```python
from build123d import *

# Parameters (mm, degrees)
SIDEBUMPERS_START       = -58.795147929
SIDEBUMPERS_OUTLINE_W   = 5.08
SIDEBUMPERS_OUTLINE_H   = 12.7
SIDEBUMPERS_DEPTH       = 21
SIDEBUMPERS_START_2     = -79.295147929
SIDEBUMPERS_2_OUTLINE_W = 5.08
SIDEBUMPERS_2_OUTLINE_H = 2.54
SIDEBUMPERS_2_DEPTH     = 62
SKETCH3_W               = 20.5
SKETCH3_H               = 5.08
CUT_EXTRUDE1_DEPTH      = 5.08
SKETCH5_W               = 21
SKETCH5_H               = 5.08
BOSS_EXTRUDE1_DEPTH     = 3
SKETCH8_W               = 41.5
SKETCH8_H               = 5.08
BOSS_EXTRUDE3_DEPTH     = 12
FILLET2_R               = 12
SKETCH9_W               = 4
SKETCH9_H               = 8.7
CUT_EXTRUDE5_DEPTH      = 5.08


# Read off the part's stored shape, not the designer's step: SideBumpers
with BuildPart() as part:
    # SideBumpers outline → SideBumpers (new body)
    with BuildSketch(Plane.YZ.offset(SIDEBUMPERS_START)):
        with Locations((-9.174171779, 10.734849265)):
            Rectangle(SIDEBUMPERS_OUTLINE_W, SIDEBUMPERS_OUTLINE_H)
    extrude(amount=SIDEBUMPERS_DEPTH)

    # SideBumpers 2 outline → SideBumpers 2 (add)
    with BuildSketch(Plane.YZ.offset(SIDEBUMPERS_START_2)):
        with Locations((-9.174171779, 5.654849265)):
            Rectangle(SIDEBUMPERS_2_OUTLINE_W, SIDEBUMPERS_2_OUTLINE_H)
    extrude(amount=SIDEBUMPERS_2_DEPTH)

    # Sketch3 → Cut-Extrude1 (cut)
    with BuildSketch(Plane(origin=(0, 0, 4.384849265), x_dir=(-1, 0, 0), z_dir=(0, 0, -1))):
        with Locations((27.545147929, -9.174171779)):
            Rectangle(SKETCH3_W, SKETCH3_H)
    extrude(amount=-CUT_EXTRUDE1_DEPTH, mode=Mode.SUBTRACT)

    # Sketch5 → Boss-Extrude1 (add)
    with BuildSketch(Plane.XY.offset(17.084849265)):
        with Locations((-48.295147929, -9.174171779)):
            Rectangle(SKETCH5_W, SKETCH5_H)
    extrude(amount=BOSS_EXTRUDE1_DEPTH)

    # Sketch8 → Boss-Extrude3 (add)
    with BuildSketch(Plane(origin=(0, 0, 4.384849265), x_dir=(-1, 0, 0), z_dir=(0, 0, -1))):
        with Locations((58.545147929, -9.174171779)):
            Rectangle(SKETCH8_W, SKETCH8_H)
    extrude(amount=BOSS_EXTRUDE3_DEPTH)

    # Fillet2
    fillet2_edges = [part.edges().sort_by_distance(p)[0] for p in [
        (-79.295147929, -9.174171779, -7.615150735),
        (-37.795147929, -9.174171779, -7.615150735),
    ]]
    fillet(fillet2_edges, radius=FILLET2_R)

    # Sketch9 → Cut-Extrude5 (cut)
    with BuildSketch(Plane(origin=(0, -6.634171779, 0), x_dir=(1, 0, 0), z_dir=(0, 1, 0))):
        with Locations((-44.128481262, -11.274849265)):
            Rectangle(SKETCH9_W, SKETCH9_H)
        with Locations((-52.461814595, -11.274849265)):
            Rectangle(SKETCH9_W, SKETCH9_H)
    extrude(amount=-CUT_EXTRUDE5_DEPTH, mode=Mode.SUBTRACT)


solid = part.part
```
Here's how the part is built. I have some questions about the finished solid (model axes, mm). A direction names the side the tool comes from. Coordinates: 2 decimals unless noted, no trailing zeros. Write each loop counter-clockwise with the first axis right and the second up, starting at its lowest first coordinate (ties: lowest second). Pieces come first, ordered by that corner, then holes. Notation, with made-up numbers: M 52,21 L 104,21 A22 cw 104,41 Z; hole C 57.5,-9 d10. An arc over 180 degrees is marked long. Answer as CSV lines item,"result". Start each with the question number.
Q1. Suppose I cut it at C-C, the plane y = -9.3. List the corners of the cut face in (x, z) for me, then the cut area to 3 significant figures.
Q2. Will these pins go through, and if not, where does the flat tip stop? pin 1 Ø3 at (x, y) = (-68.5, -10.5) entering from +Z; pin 2 Ø1.2 at (x, y) = (-44, -10) entering from -Z; pin 3 Ø2.5 at (y, z) = (-9, 11) entering from -X.
Q3. Suppose I cut it at A-A, the plane z = 14. List the corners of the cut face in (x, y) for me.
Q4. I need wall thicknesses on probe 1 along X at (y, z) = (-8.8, 10.25); probe 2 along Z at (x, y) = (-54, -10.65); probe 3 along X at (y, z) = (-9.45, 4.25). Which ranges of each line are inside material? Lowest first, please. Write a range as [from, to].
Q5. Suppose I cut it at B-B, the plane x = -52.5. List the corners of the cut face in (y, z) for me, then the cut area to 3 significant figures.
Q6. Suppose I cut it at D-D, the plane z = 18.5. List the corners of the cut face in (x, y) for me.
Q7. If we mould it in two halves opening along Z, with no side actions, what happens to faces 1 (the flat face through (-50.462, -9, 11)), 2 (the cylindrical face through (-75.87, -9.14, -4.01)), 3 (the flat face through (-58, -11.714, 3))? For each: pulls with the +Z half, pulls with the -Z half, needs draft (parallel to the pull), parting line crosses it, or undercut.
Q8. For faces 4 (the flat face through (-58.795, -9, 13)), 5 (the flat face through (-37.795, -9, 12)), 6 (the flat face through (-52, -9, 15.625)), which set-ups out of +Z, -Z, +X, -X, +Y, -Y let a thin tool reach every point of the face, with its end or its side?
Entries:
1,outline,"M -79.3,4.38 A12 ccw -67.3,-7.62 L -49.8,-7.62 A12 ccw -37.8,4.38 L -37.8,20.08 L -58.8,20.08 L -58.8,6.92 L -79.3,6.92 Z; hole M -54.46,6.92 L -50.46,6.92 L -50.46,15.62 L -54.46,15.62 Z; hole M -46.13,6.92 L -42.13,6.92 L -42.13,15.62 L -46.13,15.62 Z"
1,area,"748 mm²"
2,pin 1,"stops at z = 6.92"
2,pin 2,"stops at z = -6.43"
2,pin 3,"stops at x = -58.8"
3,outline,"M -58.8,-11.71 L -54.46,-11.71 L -54.46,-6.63 L -58.8,-6.63 Z; M -50.46,-11.71 L -46.13,-11.71 L -46.13,-6.63 L -50.46,-6.63 Z; M -42.13,-11.71 L -37.8,-11.71 L -37.8,-6.63 L -42.13,-6.63 Z"
4,probe 1,"x = [-58.8, -54.46], [-50.46, -46.13], [-42.13, -37.8]"
4,probe 2,"z = [-7.62, 6.92], [15.62, 20.08]"
4,probe 3,"x = [-79.29, -37.8]"
5,outline,"M -11.71,-7.62 L -6.63,-7.62 L -6.63,6.92 L -11.71,6.92 Z; M -11.71,15.62 L -6.63,15.62 L -6.63,20.08 L -11.71,20.08 Z"
5,area,"96.5 mm²"
6,outline,"M -58.8,-11.71 L -37.8,-11.71 L -37.8,-6.63 L -58.8,-6.63 Z"
7,face 1,"undercut"
7,face 2,"pulls with the -Z half"
7,face 3,"needs draft"
8,face 4,"+Z, -X, +Y, -Y"
8,face 5,"+Z, -Z, +X, +Y, -Y"
8,face 6,"+Y, -Y"
